Here's how the part is built. I have some questions about the finished solid (model axes, mm). A direction names the side the tool comes from. Give positions to 0.01 mm unless a question says otherwise; leave off trailing zeros. Write each loop counter-clockwise with the first axis right and the second up, starting at its lowest first coordinate (ties: lowest second). Pieces come first, ordered by that corner, then holes. Notation, with made-up numbers: (2.5, -1) - (40.5, -1) arc R10 cw to (40.5, 7) - close; hole circle Ø8 at (86, -28). An arc over 180 degrees is marked (long way). One line per item, written item: value. Start each with the question number.
1) Please list where these lines run through material, in increasing order: L1, parallel to Z at x = -3.7, y = 1.25; L2, parallel to Z at x = -29.5, y = -18.5; L3, parallel to Y at x = -11, z = -41. Write a range as [from, to].
2) On a 3-axis mill with a long thin cutter (end or side, diameter ignored), from which of +Z, -Z, +X, -X, +Y, -Y can I reach the whole of each face in a straight line? I mean faces 1 (the flat face through (-6, 0, -8)), 2 (the flat face through (-1, 3, -59)), 3 (the flat face through (-15, -18, -43)), 4 (the flat face through (-25, -15, -38)). Say none if no direction works.
3) I'm going to push flat-ended pins straight in: P1, Ø0.6, axis at y = 11, z = -28.5, coming from the -X side; P2, Ø3, axis at y = -13.5, z = -18.5, coming from the -X side; P3, Ø10, axis at y = -75.5, z = -54.5, coming from the -X side; P4, Ø5, axis at x = -22, y = -19.5, coming from the +Z side. Where does each tip first touch, or does it pass through?
4) We'd pull the mould along X, two halves only. Please class faces 5 (the cylindrical face through (-7.45, 1.48, -11.39)), 6 (the flat face through (-9.5, 1, -32)), 7 (the cylindrical face through (-20.28, -56.596, -45.177)), 8 (the cylindrical face through (-7.45, 1.48, -59.39)): +X half, -X half, draft (parallel to the pull), parting line (faces both ways), or undercut.
5) Imagine slicing it at D-D on z = -25. Write out the boundary of the cut face in (x, y), plus the area to 3 significant figures.
6) Imagine slicing it at B-B on x = -3.7. Write out the boundary of the cut face in (y, z), plus the area to 3 significant figures.
7) Imagine slicing it at C-C on x = -16.5. Write out the boundary of the cut face in (y, z).
8) Imagine slicing it at A-A on z = -11.5. Write out the boundary of the cut face in (x, y), plus the area to 3 significant figures.
Autodesk Inventor part; units mm, degrees
ref_plane "YZ Plane" through (0, 0, 0) normal (1, 0, 0) x (0, 1, 0)
ref_plane "XZ Plane" through (0, 0, 0) normal (0, 1, 0) x (-1, 0, 0)
ref_plane "XY Plane" through (0, 0, 0) normal (0, 0, 1) x (1, 0, 0)
sketch "Sketch1" plane through (0, 0, 0) normal (0, 1, 0) x (-1, 0, 0)
  line L0 (0, 0) -> (9.5, 0)
  line L1 (9.5, 0) -> (9.5, -64)
  line L2 (9.5, -64) -> (0, -64)
  line L3 (0, -64) -> (0, 0)
  circle A0 centre (3.7, -11.5) radius 2.25
  circle A1 centre (3.7, -59.5) radius 2.25
  line L4 (3.7, -11.5) -> (3.7, -59.5) construction
  dimension "d1" = 9.5
  dimension "d2" = 64
  dimension "d3" = 4.5
  dimension "d4" = 48
  dimension "d6" = 3.7
  dimension "d17" = 4.5
extrude "Extrusion1" add sketch "Sketch1" along normal blind 12
sketch "Sketch2" plane through (-9.5, 0, 0) normal (0, 0, 1) x (1, 0, 0)
  line L0 (9.5, 12) -> (0, 12)
  line L1 (3, 12) -> (8.4, 12)
  line L2 (8.4, 12) -> (8.4, 10.8)
  line L3 (8.4, 10.8) -> (3, 10.8)
  line L4 (3, 10.8) -> (3, 12)
  line L5 (9.5, 0) -> (9.5, 12)
  line L6 (3.55, 0) -> (8.05, 0)
  line L7 (3.55, 12) -> (8.05, 12)
  line L8 (9.5, 0) -> (9.5, 12)
  line L9 (9.5, 0) -> (9.5, 12)
  line L10 (3.55, 12) -> (8.05, 12)
  line L11 (3.55, 12) -> (3.55, 0)
  line L12 (3.55, 12) -> (8.05, 12)
  line L13 (3.55, 0) -> (8.05, 0)
  line L14 (3.55, 12) -> (8.05, 12)
  line L15 (3.55, 0) -> (8.05, 0)
  line L16 (3.55, 12) -> (8.05, 12)
  line L17 (3.55, 0) -> (8.05, 0)
  dimension "d9" = 1.1
  dimension "d10" = 5.4
  dimension "d11" = 1.2
  dimension "d76" = 12
extrude "Extrusion2" cut sketch "Sketch2" against normal up to next
sketch "Sketch3" plane through (0, 0, 0) normal (0, -1, 0) x (1, 0, 0)
  circle A0 centre (-3.7, -11.5) radius 2.25
  circle A1 centre (-3.7, -11.5) radius 3.75
  circle A2 centre (-3.7, -59.5) radius 2.25
  circle A3 centre (-3.7, -59.5) radius 3.75
  point P0 (0, 0)
  dimension "d14" = 7.5
extrude "Extrusion3" cut sketch "Sketch3" against normal blind 3
fillet "Fillet1" radius 1 4 edges at (0, 1.5, -58.8897) (0, 1.5, -60.1103) (0, 1.5, -10.8897) (0, 1.5, -12.1103)
fillet "Fillet2" radius 4 2 edges at (-9.5, 6, -64) (-9.5, 6, 0)
sketch "Sketch15" plane through (0, 0, 0) normal (0, -1, 0) x (1, 0, 0)
  line L0 (0, 0) -> (0, -7.592)
  line L1 (-9.5, -32) -> (-9.5, -21)
  line L2 (-9.5, -21) -> (0, -21)
  line L3 (0, -21) -> (0, -43)
  line L4 (0, -43) -> (-9.5, -43)
  line L5 (-9.5, -43) -> (-9.5, -32)
  dimension "d79" = 11
  dimension "d80" = 22
extrude "Extrusion15" add sketch "Sketch15" along normal blind 15
sketch "Sketch16" plane through (0, -15, 0) normal (0, -1, 0) x (1, 0, 0)
  line L0 (0, -43) -> (-9.5, -43)
  line L1 (0, -43) -> (-40, -43)
  line L2 (-40, -43) -> (-40, -33)
  line L3 (-40, -33) -> (0, -33)
  line L4 (0, -33) -> (0, -43)
  point P0 (0, 0)
  dimension "d83" = 40
  dimension "d84" = 10
extrude "Extrusion16" add sketch "Sketch16" along normal blind 10
sketch "Sketch17" plane through (0, -25, 0) normal (0, -1, 0) x (1, 0, 0)
  line L0 (0, -33) -> (0, -21)
  line L1 (-40, -43) -> (-9.5, -43)
  line L2 (0, -33) -> (-40, -33)
  line L3 (-40, -33) -> (-40, -43)
  line L4 (-40, -43) -> (0, -43)
  line L5 (0, -43) -> (0, -33)
  point P0 (0, 0)
  point P1 (-9.5, -43)
sketch "Sketch18" plane through (-40, -15, -43) normal (-1, 0, 0) x (0, 0, 1)
  line L0 (0, -10) -> (10, -10)
  arc A0 (5, -10) -> (5, -80) centre (53.734, -45) ccw
  point P0 (43, 15)
  dimension "d87" = 70
  dimension "d88" = 60
sweep "Sweep1" add profiles "Sketch17" path "Sketch18" path curves A0
properties part number "Back"
Numbers:
1. L1: [-64, -63.25], [-55.75, -15.25], [-7.75, 0]
1. L2: [-43, -33]
1. L3: [-97.89, -81.48], [-38.52, -15]
2. face 1: +Z, +X, -X, -Y
2. face 2: -Y
2. face 3: -Z, +X, -X
2. face 4: +Z, -Z, -X, +Y
3. P1: x = -9.5
3. P2: through
3. P3: x = -40
3. P4: z = -33
4. face 5: undercut
4. face 6: -X half
4. face 7: draft
4. face 8: undercut
5. outline: (-9.5, -15) - (0, -15) - (0, 12) - (-1.1, 12) - (-1.1, 10.8) - (-6.5, 10.8) - (-6.5, 12) - (-9.5, 12) - close
5. area: 250 mm^2
6. outline: (-99.74, -39.6) arc R64.13 ccw to (-25, -43) - (0, -43) - (0, -55.75) - (3, -55.75) - (3, -57.25) - (10.8, -57.25) - (10.8, -13.75) - (3, -13.75) - (3, -15.25) - (0, -15.25) - (0, -21) - (-15, -21) - (-15, -33) - (-25, -33) arc R56.01 cw to (-90.26, -36.4) - close; (0, -64) - (10.8, -64) - (10.8, -61.75) - (3, -61.75) - (3, -63.25) - (0, -63.25) - close; (0, -7.75) - (3, -7.75) - (3, -9.25) - (10.8, -9.25) - (10.8, 0) - (0, 0) - close
6. area: 1,610 mm^2
7. outline: (-99.74, -39.6) arc R64.13 ccw to (-25, -43) - (-15, -43) - (-15, -33) - (-25, -33) arc R56.01 cw to (-90.26, -36.4) - close
8. outline: (-9.5, 0) - (-7.45, 0) - (-7.45, 3) - (-5.95, 3) - (-5.95, 10.8) - (-6.5, 10.8) - (-6.5, 12) - (-9.5, 12) - close; (-1.45, 3) - (0, 3) - (0, 12) - (-1.1, 12) - (-1.1, 10.8) - (-1.45, 10.8) - close
8. area: 50.1 mm^2
